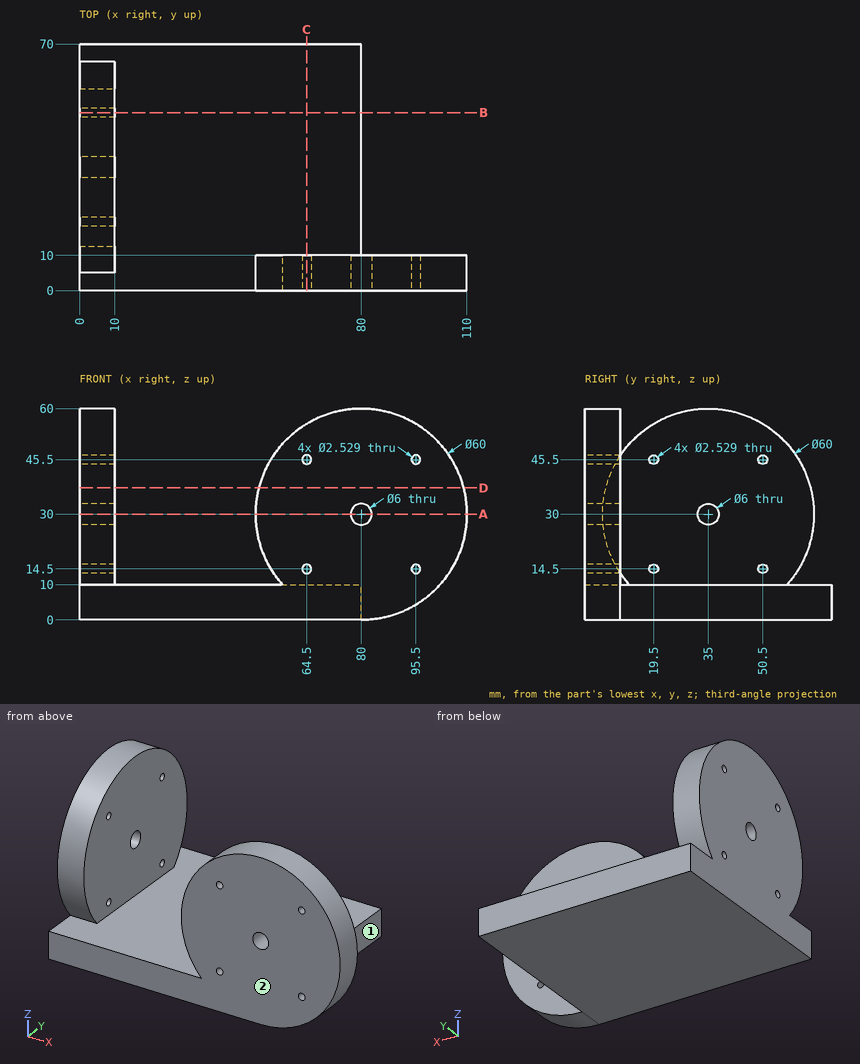
Geometry: see drawing. Coordinates: mm, zero at the bounding-box minimum. A direction names the side the tool comes from. Round coordinates to 2 decimals unless told otherwise and drop trailing zeros. Loops run counter-clockwise (first coordinate to the right, second up) from the corner with the lowest first, then second, coordinate; pieces in that order, holes last. Notation, with made-up numbers: M 47,-21.75 L 95,-21.75 A22 cw 95,5.25 Z; hole C 17.5,-19 d11. An arc over 180 degrees is marked long. Use a Markdown table: item, result. Add a question column.
1. Ray query, line 1 along X through (y, z) = (7, 30); line 2 along Y through (x, z) = (6, 30); line 3 along Y through (x, z) = (7, 45.5). Return the intervals inside material, ascending. Write a range as [from, to].
2. Cut plane D-D, the plane z = 37.5. Output: boundary loops of the cut face in (x, y).
3. Contact query for flat-ended pins moving along their axis: pin 1 (1.5 mm diameter, centred on x = 92.5, z = 52, fed in from -Y); pin 2 (3 mm diameter, centred on y = 42.5, z = 36.5, fed in from +X); pin 3 (3 mm diameter, centred on x = 64.5, z = 45.5, fed in from +Y); pin 4 (21 mm diameter, centred on x = 50.5, y = 43.5, fed in from +Z). Output: stop coordinate, or through.
4. Cut plane B-B, the plane y = 50.5. Output: boundary loops of the cut face in (x, z).
5. Cut plane A-A, the plane z = 30. Output: boundary loops of the cut face in (x, y), and give its area (3 significant figures).
6. Set-up query: the marked faces 1 and 2. Return all of +Z, -Z, +X, -X, +Y, -Y with unobstructed straight access to the full face (end or side cutting, diameter ignored); none if empty.
7. Cut plane C-C, the plane x = 64.5. Output: boundary loops of the cut face in (y, z).
Solution:
| question | item | result |
|---|---|---|
| 1 | line 1 | x = [0, 10], [50, 77], [83, 110] |
| 1 | line 2 | y = [5, 32], [38, 65] |
| 1 | line 3 | y = [9.31, 18.24], [20.76, 49.24], [51.76, 60.69] |
| 2 | outline | M 0,5.95 L 10,5.95 L 10,64.05 L 0,64.05 Z; M 50.95,0 L 109.05,0 L 109.05,10 L 50.95,10 Z |
| 3 | pin 1 | stops at y = 0 |
| 3 | pin 2 | stops at x = 10 |
| 3 | pin 3 | stops at y = 10 |
| 3 | pin 4 | stops at z = 10 |
| 4 | outline | M 0,0 L 80,0 L 80,10 L 10,10 L 10,13.24 L 0,13.24 Z; M 0,15.76 L 10,15.76 L 10,44.24 L 0,44.24 Z; M 0,46.76 L 10,46.76 L 10,55.69 L 0,55.69 Z |
| 5 | outline | M 0,5 L 10,5 L 10,32 L 0,32 Z; M 0,38 L 10,38 L 10,65 L 0,65 Z; M 50,0 L 77,0 L 77,10 L 50,10 Z; M 83,0 L 110,0 L 110,10 L 83,10 Z |
| 5 | area | 1,080 mm2 |
| 6 | face 1 | +Z, -Z, +X, +Y |
| 6 | face 2 | +Z, -Z, +X, -X, -Y |
| 7 | outline | M 0,0 L 70,0 L 70,10 L 10,10 L 10,13.24 L 0,13.24 Z; M 0,15.76 L 10,15.76 L 10,44.24 L 0,44.24 Z; M 0,46.76 L 10,46.76 L 10,55.69 L 0,55.69 Z |
